Study the drawing (mm; zero at the part's minimum x, y, z) and answer. A direction names the side the tool comes from. Round coordinates to 2 decimals unless told otherwise and drop trailing zeros. Write each loop counter-clockwise with the first axis right and the second up, starting at its lowest first coordinate (ties: lowest second). Pieces come first, ordered by that corner, then holes. Notation, with made-up numbers: (31.5, 1.5) - (52.5, 1.5) arc R22 ccw to (52.5, 23.5) - close; hole circle Ø7 at (33.5, 85). An arc over 180 degrees is marked (long way). Use one line per item in the form item = value. Start each with the question number.
1) For the marked faces 4 and 5, determine the directions among +Z, -Z, +X, -X, +Y, -Y from which every point of the face is accessible in a straight line to the end or side of a thin tool.
2) The part is cut by section A-A, the plane z = 68. Give the vertices of the cut face in (x, y), plus the area to 3 significant figures.
3) The part is cut by section B-B, the plane y = 63.5. Give the vertices of the cut face in (x, z), plus the area to 3 significant figures.
4) Consider line 1 along Y through (x, z) = (63.5, 74.75); line 2 along Z through (x, y) = (49.5, 89.5). Determine where each line is inside the solid, lowest interval first. Write a range as from..to.
5) Each of these flat-tipped pins is pushed along its axis until it touches: pin 1 (4 mm diameter, centred on x = 51, y = 72, fed in from -Z); pin 2 (10 mm diameter, centred on x = 37, y = 92, fed in from +Z). Where does it stop, or does it pass through?
6) For a pull along Y with two mould halves and no side action, classify the marked faces 1, 2 and 3 as released by +Y, released by -Y, zero draft, split by the parting line, or undercut.
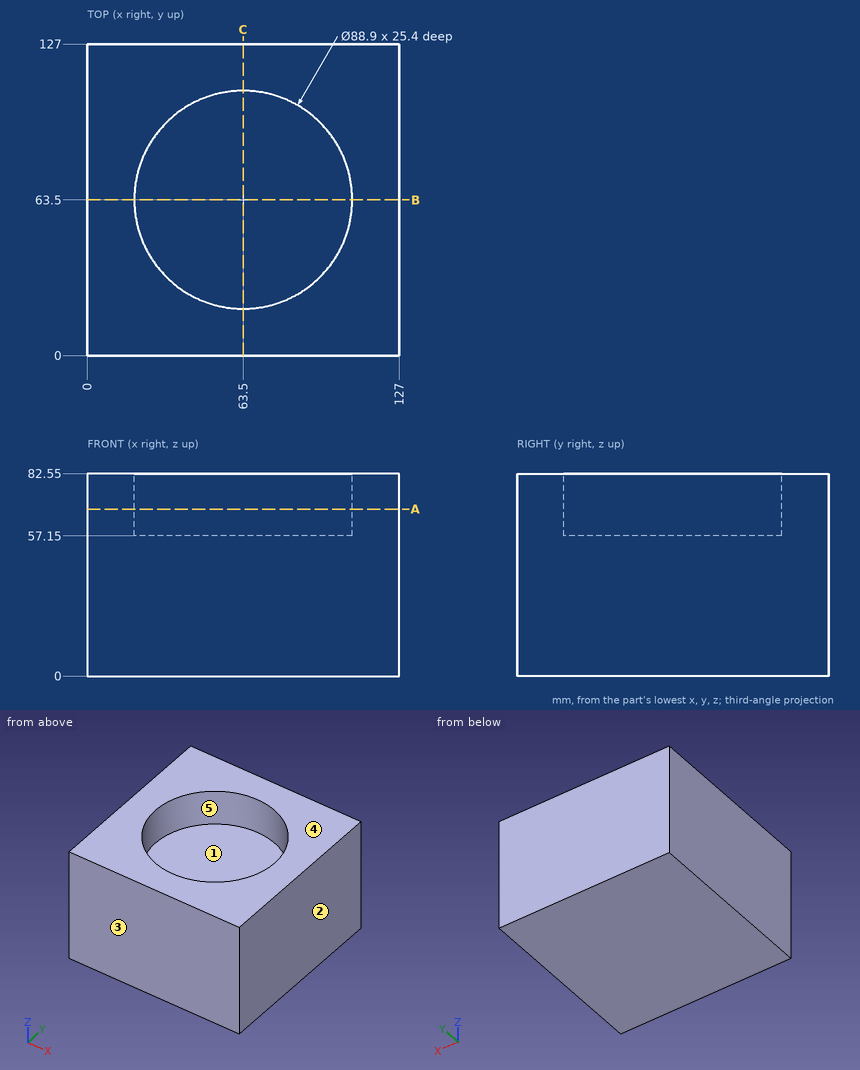
Geometry results:
q1.face_4 = +Z, +X, -X, +Y, -Y
q1.face_5 = +Z
q2.outline = (0, 0) - (127, 0) - (127, 127) - (0, 127) - close; hole circle Ø88.9 at (63.5, 63.5)
q2.area = 9,920 mm2
q3.outline = (0, 0) - (127, 0) - (127, 82.55) - (107.95, 82.55) - (107.95, 57.15) - (19.05, 57.15) - (19.05, 82.55) - (0, 82.55) - close
q3.area = 8,230 mm2
q4.line_1 = 0..19.05, 107.95..127
q4.line_2 = 0..57.15
q5.pin_1 = 0
q5.pin_2 = 57.15
q6.face_1 = undercut
q6.face_2 = zero draft
q6.face_3 = released by -Y
